CAD build for the part. Positions are in the model's coordinates, mm. Face numbers are marked on the shaded views. A direction names the side the tool comes from. Round coordinates to 2 decimals unless told otherwise and drop trailing zeros. Write each loop counter-clockwise with the first axis right and the second up, starting at its lowest first coordinate (ties: lowest second). Pieces come first, ordered by that corner, then holes. Notation, with made-up numbers: (31.25, 49.5) - (52.25, 49.5) arc R17 ccw to (52.25, 66.5) - close; hole circle Ø6 at (17, 21.5). An arc over 180 degrees is marked (long way). Answer in a Markdown table with one row per item.
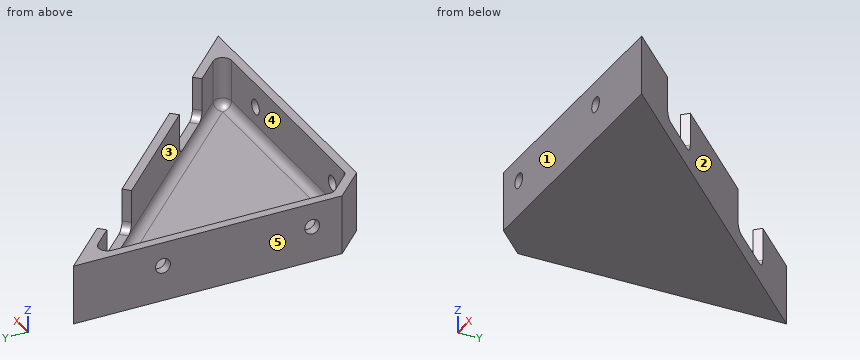
```python
from build123d import *

# Parameters (mm, degrees)
F1_DEPTH  = 20
F2_SIZE   = 10
F3_T      = -3
F5_R      = 2.5
F6_DEPTH  = 3
F4_R      = 2.5
F7_DEPTH  = 3
F9_R      = 3
F10_DEPTH = 3


with BuildPart() as f1:
    # F0 (on Top) → F1 (new body)
    with BuildSketch(Plane.XY):
        Polygon((0, 100), (0, 0), (100, 0), align=None)
    extrude(amount=F1_DEPTH)

    # F2
    f2_edges = [f1.edges().sort_by_distance(p)[0] for p in [
        (0, 0, 10),
    ]]
    chamfer(f2_edges, length=F2_SIZE)

    # F3
    f3_openings = [f1.faces().sort_by_distance(p)[0] for p in [
        (33.636364, 33.636364, 20),
    ]]
    offset(amount=F3_T, openings=f3_openings)

    # F5 (on Front) → F6 (cut, through all)
    with BuildSketch(Plane.XZ):
        with Locations((20, 12)):
            Circle(F5_R)
        with Locations((70, 12)):
            Circle(F5_R)
    extrude(amount=-F6_DEPTH, mode=Mode.SUBTRACT)

    # F4 (on Right) → F7 (cut, through all)
    with BuildSketch(Plane.YZ):
        with Locations((20, 12)):
            Circle(F4_R)
        with Locations((70, 12)):
            Circle(F4_R)
    extrude(amount=F7_DEPTH, mode=Mode.SUBTRACT)

    # F9
    f9_edges = [f1.edges().sort_by_distance(p)[0] for p in [
        (3, 52, 3),
        (52, 3, 3),
        (92.757359, 3, 11.5),
        (3, 92.757359, 11.5),
        (47.87868, 47.87868, 3),
        (3, 11.242641, 11.5),
        (11.242641, 3, 11.5),
    ]]
    fillet(f9_edges, radius=F9_R)

    # F8 (on face) → F10 (cut, through all)
    with BuildSketch(Plane(origin=(50, 50, 0), x_dir=(-0.7071067812, 0.7071067812, 0), z_dir=(0.7071067812, 0.7071067812, 0))):
        with BuildLine():
            Line((-23.2842712475, 20), (-45.4264068712, 20))
            Line((-45.4264068712, 20), (-45.4264068712, 9))
            ThreePointArc((-45.4264068712, 9), (-44.5477272148, 6.8786796564), (-42.4264068712, 6))
            Line((-42.4264068712, 6), (-26.2842712475, 6))
            ThreePointArc((-26.2842712475, 6), (-24.1629509039, 6.8786796564), (-23.2842712475, 9))
            Line((-23.2842712475, 9), (-23.2842712475, 20))
        make_face()
        with BuildLine():
            Line((47.4264068712, 20), (23.2842712475, 20))
            Line((23.2842712475, 20), (23.2842712475, 9))
            ThreePointArc((23.2842712475, 9), (24.1629509039, 6.8786796564), (26.2842712475, 6))
            Line((26.2842712475, 6), (44.4264068712, 6))
            ThreePointArc((44.4264068712, 6), (46.5477272148, 6.8786796564), (47.4264068712, 9))
            Line((47.4264068712, 9), (47.4264068712, 20))
        make_face()
    extrude(amount=-F10_DEPTH, mode=Mode.SUBTRACT)


solid = f1.part
```
Q1. Flat gauge pins, fed straight in: pin 1 (16.5 mm diameter, centred on x = 21, y = 72.5, fed in from +Z); pin 2 (4.5 mm diameter, centred on y = 20, z = 12, fed in from +X); pin 3 (4 mm diameter, centred on y = 54.5, z = 13.5, fed in from +X); pin 4 (4 mm diameter, centred on x = 20, z = 12, fed in from +Y). Where does each tip first touch, or does it go through?
Computed:
| item | result |
|---|---|
| pin 1 | stops at z = 6 |
| pin 2 | stops at x = 82.25 |
| pin 3 | stops at x = 47.5 |
| pin 4 | passes through |
Q2. 3-axis set-ups, long thin cutter, end or side, ignore diameter. For the marked faces 4 and 5: which of +Z, -Z, +X, -X, +Y, -Y reach the whole face in a straight line?
Computed:
| item | result |
|---|---|
| face 4 | +Z |
| face 5 | +Z, -Z, -X, +Y, -Y |
Q3. Pull direction X, two halves, no side cores. Call the marked faces 1, 2 and 3: released by +X, released by -X, zero draft, split by the parting line, or undercut.
Computed:
| item | result |
|---|---|
| face 1 | zero draft |
| face 2 | released by +X |
| face 3 | undercut |
Q4. Saw through at B-B on z = 12. Count the separate pieces of the cut face and the enclosed holes in it, then the cut area to 3 significant figures.
Computed:
| item | result |
|---|---|
| separate pieces | 6 |
| enclosed holes | 0 |
| area | 780 mm2 |
Q5. Drill centre lines: line 1 (Z direction, x = 1.2, y = 70); line 2 (Y direction, x = 28, z = 9); line 3 (Y direction, x = 31, z = 5). Where is each one in solid material? Low to high.
Computed:
| item | result |
|---|---|
| line 1 | z = 0 to 9.5, 14.5 to 20 |
| line 2 | y = 0 to 3 |
| line 3 | y = 0 to 3.17, 64.51 to 69 |
Q6. Saw through at A-A on z = 17.5. List the corners of the cut face in (x, y).
Computed:
| item | result |
|---|---|
| outline | (0, 10) - (10, 0) - (100, 0) - (82.12, 17.88) - (80, 15.76) - (87.64, 8.12) arc R3 cw to (85.51, 3) - (12.49, 3) arc R3 cw to (10.36, 3.88) - (3.88, 10.36) arc R3 cw to (3, 12.49) - (3, 85.51) arc R3 cw to (8.12, 87.64) - (14.34, 81.41) - (16.46, 83.54) - (0, 100) - close; (31.41, 64.34) - (64.34, 31.41) - (66.46, 33.54) - (33.54, 66.46) - close |
